Can you work these out from the model? Positions are in its coordinate system, mm. A direction names the side the tool comes from. Give positions to 0.01 mm unless a question says otherwise; leave off trailing zeros. Order: outer loops, then holes, each group sorted by start corner. A loop starts at its lowest first (then second) coordinate and runs counter-clockwise, first axis right, second up. Notation, with made-up numbers: (11.5, 86) - (40.5, 86) arc R23 ccw to (40.5, 98) - close; hole circle Ø11 at (65.25, 87.25). An arc over 180 degrees is marked (long way). Answer as a JSON object with one key per item and string values.
```python
from build123d import *

# Parameters (mm, degrees)
SKETCH1_W           = 64
SKETCH1_H           = 84
BOSS_EXTRUDE1_DEPTH = 3
BOSS_EXTRUDE2_DEPTH = 1
SKETCH3_R           = 2.1
BOSS_EXTRUDE3_DEPTH = 3
FILLET3_R           = 5
FILLET4_R           = 2
CUT_EXTRUDE1_DEPTH  = 10


with BuildPart() as part:
    # Sketch1 → Boss-Extrude1 (new body)
    with BuildSketch(Plane(origin=(0, 0, 0), x_dir=(1, 0, 0), z_dir=(0, 1, 0))):
        with Locations((32, -42)):
            Rectangle(SKETCH1_W, SKETCH1_H)
    extrude(amount=BOSS_EXTRUDE1_DEPTH)

    # Sketch2 → Boss-Extrude2 (add)
    with BuildSketch(Plane(origin=(0, 3, 0), x_dir=(1, 0, 0), z_dir=(0, 1, 0))):
        Polygon((23.75, -68.961175578), (23.75, -78), (46.25, -78), (46.25, -68.961175578), (46.25, -38.961175578), (48.25, -38.961175578), (48.25, -80), (21.75, -80), (21.75, -38.961175578), (23.75, -38.961175578), align=None)
    extrude(amount=BOSS_EXTRUDE2_DEPTH)


with BuildPart() as body_2:
    # Sketch3 → Boss-Extrude3 (new body)
    # profile 1 of 10: a face of its own
    with BuildSketch(Plane(origin=(0, 3, 0), x_dir=(1, 0, 0), z_dir=(0, 1, 0))):
        with BuildLine():
            Line((0, -76.928932188), (-7.778174593, -84.707106781))
            ThreePointArc((-7.778174593, -84.707106781), (-4.242640687, -83.242640687), (-0.707106781, -84.707106781))
            ThreePointArc((-0.707106781, -84.707106781), (0.376756975, -86.329223525), (0.757359313, -88.242640687))
            ThreePointArc((0.757359313, -88.242640687), (0.391358456, -90.120419145), (-0.653061462, -91.723290194))
            Line((-0.653061462, -91.723290194), (7.070228732, -84))
            Line((7.070228732, -84), (0, -84))
            Line((0, -84), (0, -76.928932188))
        make_face()
    # profile 2 of 10: a face of its own
    with BuildSketch(Plane(origin=(0, 3, 0), x_dir=(1, 0, 0), z_dir=(0, 1, 0))):
        with BuildLine():
            ThreePointArc((-0.707106781, -84.707106781), (-4.242640687, -83.242640687), (-7.778174593, -84.707106781))
            Line((-7.778174593, -84.707106781), (-0.707106781, -84.707106781))
        make_face()
    # profile 3 of 10: a face of its own
    with BuildSketch(Plane(origin=(0, 3, 0), x_dir=(1, 0, 0), z_dir=(0, 1, 0))):
        with BuildLine():
            ThreePointArc((0.757359313, -88.242640687), (0.376756975, -86.329223525), (-0.707106781, -84.707106781))
            Line((-0.707106781, -84.707106781), (-0.76199118, -91.832219912))
            Line((-0.76199118, -91.832219912), (-0.653061462, -91.723290194))
            ThreePointArc((-0.653061462, -91.723290194), (0.391358456, -90.120419145), (0.757359313, -88.242640687))
        make_face()
    # profile 4 of 10: a face of its own
    with BuildSketch(Plane(origin=(0, 3, 0), x_dir=(1, 0, 0), z_dir=(0, 1, 0))):
        with BuildLine():
            Line((-0.707106781, -84.707106781), (-7.778174593, -84.707106781))
            ThreePointArc((-7.778174593, -84.707106781), (-7.805302944, -91.750836469), (-0.76199118, -91.832219912))
            Line((-0.76199118, -91.832219912), (-0.707106781, -84.707106781))
        make_face()
        with Locations(Location((-4.242640687, -88.242640687, 0), (0, 0, 270))):
            Circle(SKETCH3_R, mode=Mode.SUBTRACT)
    # profile 5 of 10: a face of its own
    with BuildSketch(Plane(origin=(0, 3, 0), x_dir=(1, 0, 0), z_dir=(0, 1, 0))):
        with BuildLine():
            Line((64.707106781, 7.778174593), (56.928932188, 0))
            Line((56.928932188, 0), (64, 0))
            Line((64, 0), (64, -7.071067812))
            Line((64, -7.071067812), (71.778174593, 0.707106781))
            ThreePointArc((71.778174593, 0.707106781), (68.242640687, -0.757359313), (64.707106781, 0.707106781))
            ThreePointArc((64.707106781, 0.707106781), (63.242640687, 4.242640687), (64.707106781, 7.778174593))
        make_face()
    # profile 6 of 10: a face of its own
    with BuildSketch(Plane(origin=(0, 3, 0), x_dir=(1, 0, 0), z_dir=(0, 1, 0))):
        with BuildLine():
            ThreePointArc((64.707106781, 0.707106781), (68.242640687, -0.757359313), (71.778174593, 0.707106781))
            Line((71.778174593, 0.707106781), (64.707106781, 0.707106781))
        make_face()
    # profile 7 of 10: a face of its own
    with BuildSketch(Plane(origin=(0, 3, 0), x_dir=(1, 0, 0), z_dir=(0, 1, 0))):
        with BuildLine():
            Line((64.707106781, 0.707106781), (64.707106781, 7.778174593))
            ThreePointArc((64.707106781, 7.778174593), (63.242640687, 4.242640687), (64.707106781, 0.707106781))
        make_face()
    # profile 8 of 10: a face of its own
    with BuildSketch(Plane(origin=(0, 3, 0), x_dir=(1, 0, 0), z_dir=(0, 1, 0))):
        with BuildLine():
            ThreePointArc((73.242640687, 4.242640687), (70.156057849, 8.86203835), (64.707106781, 7.778174593))
            Line((64.707106781, 7.778174593), (64.707106781, 0.707106781))
            Line((64.707106781, 0.707106781), (71.778174593, 0.707106781))
            ThreePointArc((71.778174593, 0.707106781), (72.86203835, 2.329223525), (73.242640687, 4.242640687))
        make_face()
        with Locations(Location((68.242640687, 4.242640687, 0), (0, 0, 270))):
            Circle(SKETCH3_R, mode=Mode.SUBTRACT)
    # profile 9 of 10: a face of its own
    with BuildSketch(Plane(origin=(0, 3, 0), x_dir=(1, 0, 0), z_dir=(0, 1, 0))):
        Polygon((7.070228732, -84), (0, -76.928932188), (0, -84), align=None)
    # profile 10 of 10: a face of its own
    with BuildSketch(Plane(origin=(0, 3, 0), x_dir=(1, 0, 0), z_dir=(0, 1, 0))):
        Polygon((64, 0), (56.928932188, 0), (64, -7.071067812), align=None)
    extrude(amount=-BOSS_EXTRUDE3_DEPTH)

    # Combine2: union part
    add(part.part)

    # Fillet3
    fillet3_edges = [body_2.edges().sort_by_distance(p)[0] for p in [
        (0, 1.5, 76.928932188),
        (7.070228732, 1.5, 84),
        (64, 1.5, 7.071067812),
        (56.928932188, 1.5, 0),
    ]]
    fillet(fillet3_edges, radius=FILLET3_R)

    # Fillet4
    fillet4_edges = [body_2.edges().sort_by_distance(p)[0] for p in [
        (64, 1.5, 84),
        (0, 1.5, 0),
    ]]
    fillet(fillet4_edges, radius=FILLET4_R)

    # Sketch4 → Cut-Extrude1 (cut)
    with BuildSketch(Plane(origin=(0, 3, 0), x_dir=(1, 0, 0), z_dir=(0, 1, 0))):
        with BuildLine():
            Line((32.95, -17.95), (32.95, -20))
            ThreePointArc((32.95, -20), (35, -22.05), (37.05, -20))
            Line((37.05, -20), (37.05, -17.95))
            ThreePointArc((37.05, -17.95), (35, -15.9), (32.95, -17.95))
        make_face()
    extrude(amount=-CUT_EXTRUDE1_DEPTH, mode=Mode.SUBTRACT)


solid = body_2.part
```
Q1. Which directions (+Z, -Z, +X, -X, +Y, -Y) give clear straight access to the entire face, cutting with the end or side of a thin tool? Please do faces 1 (the face through (32.95, 2, 19)), 2 (the face through (64, 1, 46)), 3 (the face through (0, 1, 39)).
Recorded:
{"face 1": "+Y, -Y", "face 2": "+Z, +X, +Y, -Y", "face 3": "-Z, -X, +Y, -Y"}
Q2. If we section it at B-B, the plane y = 2.35: Please give me the cut outline in (x, z).
Recorded:
{"outline": "(-7.78, 84.71) - (-1.46, 78.39) arc R5 cw to (0, 74.86) - (0, 2) arc R2 ccw to (2, 0) - (54.86, 0) arc R5 cw to (58.39, -1.46) - (64.71, -7.78) arc R5 ccw to (71.78, -0.71) - (65.46, 5.61) arc R5 cw to (64, 9.14) - (64, 82) arc R2 ccw to (62, 84) - (9.14, 84) arc R5 cw to (5.61, 85.46) - (-0.76, 91.83) arc R5 ccw to start; hole circle Ø4.2 at (-4.24, 88.24); hole (32.95, 17.95) arc R2.05 ccw to (37.05, 17.95) - (37.05, 20) arc R2.05 ccw to (32.95, 20) - close; hole circle Ø4.2 at (68.24, -4.24)"}
Q3. We'd pull the mould along Z, two halves only. Please class faces 4 (the face through (7.25, 1.48, 84.37)), 5 (the face through (37.05, 2, 19)), 6 (the face through (-4.58, 1.52, 81.51)): released by +Z, released by -Z, zero draft, split by the parting line, or undercut.
Recorded:
{"face 4": "released by +Z", "face 5": "undercut", "face 6": "released by -Z"}
Q4. If we section it at A-A, the plane x = 35: Please give me the cut outline in (y, z), then the cut area to 3 significant figures.
Recorded:
{"outline": "(0, 0) - (3, 0) - (3, 15.9) - (0, 15.9) - close; (0, 22.05) - (3, 22.05) - (3, 78) - (4, 78) - (4, 80) - (3, 80) - (3, 84) - (0, 84) - close", "area": "236 mm^2"}
Q5. I need wall thicknesses on L1, parallel to X at y = 1.6, z = 59; L2, parallel to Z at x = 45.5, y = 3.65; L3, parallel to Y at x = 39.5, z = 41.5. Which ranges of each line are inside material? Lowest first, please.
Recorded:
{"L1": "x = 0 to 64", "L2": "z = 78 to 80", "L3": "y = 0 to 3"}
Q6. I'm going to push flat-ended pins straight in: pin 1 Ø1 at (x, y) = (46.5, 1.5) entering from +Z; pin 2 Ø1 at (x, y) = (7, 1.5) entering from -Z; pin 3 Ø4 at (x, z) = (68.24, -4.24) entering from -Y; pin 4 Ø1.6 at (y, z) = (1, 19.5) entering from +X. Where does each tip first touch, or does it pass through?
Recorded:
{"pin 1": "stops at z = 84", "pin 2": "stops at z = 0", "pin 3": "passes through", "pin 4": "stops at x = 64"}
